Check sheet for the modelled part. Datum: model origin and axes. Units: mm. A direction names the side the tool comes from. Give positions to 0.01 mm unless a question says otherwise; leave off trailing zeros. Write each loop counter-clockwise with the first axis right and the second up, starting at its lowest first coordinate (ties: lowest second). Pieces come first, ordered by that corner, then holes. Notation, with made-up numbers: M 65.25,43.25 L 81.25,43.25 A24 ccw 81.25,64.25 Z; hole C -38.5,45 d6. An arc over 180 degrees is marked long. Write item = value, one per line. Start each with the question number.
1) Gauge pin test, flat ends, axial feed: pin 1 (0.7 mm diameter, centred on y = 0.5, z = -15.5, fed in from -X); pin 2 (0.8 mm diameter, centred on x = 34.5, y = 4, fed in from -Z); pin 3 (2.5 mm diameter, centred on y = 2.5, z = 2.5, fed in from -X). Record the tip position at first contact, or that the pin passes through.
2) Sectioned sample at B-B, the plane z = -7. Record the cut outline in (x, y), then the cut area to 3 significant figures.
3) Scan lines: L1, parallel to X at y = 1.6, z = 2.5; L2, parallel to X at y = 3.55, z = 7; L3, parallel to X at y = 0.9, z = -19.5. Record each from-to range of solid material in increasing order.
4) Sectioned sample at C-C, the plane x = -15.5. Record the cut outline in (y, z), then the cut area to 3 significant figures.
5) Sectioned sample at A-A, the plane x = 36.5. Record the cut outline in (y, z).
6) Set-up check for faces 4 (the face through (40.926, 3, 16)), 5 (the face through (37, 3, 4.458)), 6 (the face through (-36.274, 2, 3)), 7 (the face through (-32.274, 2, 3)): record each of +Z, -Z, +X, -X, +Y, -Y from which the full face is reachable in a straight line by a thin tool's end or side.
7) Draft check along Z on faces 1 (the face through (-2, 0, 4)), 2 (the face through (-41.324, 0.71, 14.295)), 3 (the face through (37, 3, 26.658)). Enter one of: pulls with the +Z half, pulls with the -Z half, needs draft (parallel to the pull), parting line crosses it, or undercut.
from build123d import *

# Parameters (mm, degrees)
SKETCH_1_W          = 85
SKETCH_1_H          = 56
EXTRUDE_1_DEPTH     = 1.4
FILLET_1_R          = 3
SKETCH_2_R          = 1.3
CUT_EXTRUDE_1_DEPTH = 1.5
SKETCH_7_R          = 3
CUT_EXTRUDE_4_DEPTH = 0.1
SKETCH_3_W          = 5
SKETCH_3_H          = 12.5
CUT_EXTRUDE_2_DEPTH = 1.5
FILLET_2_R          = 1
SKETCH_8_W          = 50
SKETCH_8_H          = 6.5
CUT_EXTRUDE_5_DEPTH = 54.614950043
FILLET_3_R          = 1
SKETCH_4_W          = 6.8
SKETCH_4_H          = 22
EXTRUDE_2_DEPTH     = 3.2
SKETCH_5_W          = 1.5
SKETCH_5_H          = 20.4
CUT_EXTRUDE_3_DEPTH = 1.8
SKETCH_6_W          = 4
SKETCH_6_H          = 12.5
EXTRUDE_3_DEPTH     = 2.2
SKETCH_10_R         = 2.85
EXTRUDE_4_DEPTH     = 1.4
SKETCH_9_R          = 1.85
CUT_EXTRUDE_6_DEPTH = 56.978914621
FILLET_4_R          = 1


with BuildPart() as part:
    # 草图1 → 凸台-拉伸1 (new body)
    with BuildSketch(Plane(origin=(0, 0, 0), x_dir=(1, 0, 0), z_dir=(0, 1, 0))):
        with Locations((-0.074300699, -4.558129371)):
            Rectangle(SKETCH_1_W, SKETCH_1_H)
    extrude(amount=EXTRUDE_1_DEPTH)

    # 圆角1
    fillet_1_edges = [part.edges().sort_by_distance(p)[0] for p in [
        (-42.574300699, 0.7, -23.441870629),
        (42.425699301, 0.7, -23.441870629),
        (42.425699301, 0.7, 32.558129371),
        (-42.574300699, 0.7, 32.558129371),
    ]]
    fillet(fillet_1_edges, radius=FILLET_1_R)

    # 草图2 → 切除-拉伸1 (cut)
    with BuildSketch(Plane(origin=(0, 1.4, 0), x_dir=(1, 0, 0), z_dir=(0, 1, 0))):
        with Locations(Location((-39.074300699, 19.941870629, 0), (0, 0, 270))):
            Circle(SKETCH_2_R)
        with Locations(Location((-39.074300699, -29.058129371, 0), (0, 0, 270))):
            Circle(SKETCH_2_R)
        with Locations(Location((18.925699301, -29.058129371, 0), (0, 0, 270))):
            Circle(SKETCH_2_R)
        with Locations(Location((18.925699301, 19.941870629, 0), (0, 0, 270))):
            Circle(SKETCH_2_R)
    extrude(amount=-CUT_EXTRUDE_1_DEPTH, mode=Mode.SUBTRACT)

    # 草图7 → 切除-拉伸4 (cut)
    with BuildSketch(Plane(origin=(0, 1.4, 0), x_dir=(1, 0, 0), z_dir=(0, 1, 0))):
        with Locations(Location((-39.074300699, 19.941870629, 0), (0, 0, 270))):
            Circle(SKETCH_7_R)
        with Locations(Location((18.925699301, 19.941870629, 0), (0, 0, 270))):
            Circle(SKETCH_7_R)
        with Locations(Location((-39.074300699, -29.058129371, 0), (0, 0, 270))):
            Circle(SKETCH_7_R)
        with Locations(Location((18.925699301, -29.058129371, 0), (0, 0, 270))):
            Circle(SKETCH_7_R)
    extrude(amount=-CUT_EXTRUDE_4_DEPTH, mode=Mode.SUBTRACT)

    # 草图3 → 切除-拉伸2 (cut)
    with BuildSketch(Plane(origin=(0, 1.4, 0), x_dir=(1, 0, 0), z_dir=(0, 1, 0))):
        with Locations((-40.074300699, -2.808129371)):
            Rectangle(SKETCH_3_W, SKETCH_3_H)
    extrude(amount=-CUT_EXTRUDE_2_DEPTH, mode=Mode.SUBTRACT)

    # 圆角2
    fillet_2_edges = [part.edges().sort_by_distance(p)[0] for p in [
        (-42.574300699, 0.7, 9.058129371),
        (-42.574300699, 0.7, -3.441870629),
        (-37.574300699, 0.7, -3.441870629),
        (-37.574300699, 0.7, 9.058129371),
    ]]
    fillet(fillet_2_edges, radius=FILLET_2_R)

    # 草图8 → 切除-拉伸5 (cut, through all)
    with BuildSketch(Plane(origin=(0, 1.4, 0), x_dir=(1, 0, 0), z_dir=(0, 1, 0))):
        with Locations((-10.074300699, 20.191870629)):
            Rectangle(SKETCH_8_W, SKETCH_8_H)
    extrude(amount=-CUT_EXTRUDE_5_DEPTH, mode=Mode.SUBTRACT)

    # 圆角3
    fillet_3_edges = [part.edges().sort_by_distance(p)[0] for p in [
        (-35.074300699, 0.7, -16.941870629),
        (-35.074300699, 0.7, -23.441870629),
        (14.925699301, 0.7, -23.441870629),
        (14.925699301, 0.7, -16.941870629),
    ]]
    fillet(fillet_3_edges, radius=FILLET_3_R)

    # 草图4 → 凸台-拉伸2 (add)
    with BuildSketch(Plane(origin=(0, 1.4, 0), x_dir=(1, 0, 0), z_dir=(0, 1, 0))):
        with Locations((37.525699301, 6.541870629)):
            Rectangle(SKETCH_4_W, SKETCH_4_H)
        with Locations((37.525699301, -15.658129371)):
            Rectangle(SKETCH_4_W, SKETCH_4_H)
    extrude(amount=EXTRUDE_2_DEPTH)

    # 草图5 → 切除-拉伸3 (cut)
    with BuildSketch(Plane(origin=(0, 4.6, 0), x_dir=(1, 0, 0), z_dir=(0, 1, 0))):
        with Locations((34.875699301, 6.541870629)):
            Rectangle(SKETCH_5_W, SKETCH_5_H)
        with Locations((34.875699301, -15.658129371)):
            Rectangle(SKETCH_5_W, SKETCH_5_H)
    extrude(amount=-CUT_EXTRUDE_3_DEPTH, mode=Mode.SUBTRACT)

    # 草图6 → 凸台-拉伸3 (add)
    with BuildSketch(Plane(origin=(0, 1.4, 0), x_dir=(1, 0, 0), z_dir=(0, 1, 0))):
        with Locations((-34.274300699, -2.808129371)):
            Rectangle(SKETCH_6_W, SKETCH_6_H)
    extrude(amount=EXTRUDE_3_DEPTH)

    # 草图10 → 凸台-拉伸4 (add)
    with BuildSketch(Plane(origin=(0, 1.4, 0), x_dir=(1, 0, 0), z_dir=(0, 1, 0))):
        with Locations((-42.574300699, 6.541870629)):
            Circle(SKETCH_10_R)
        with Locations((-42.574300699, -15.658129371)):
            Circle(SKETCH_10_R)
    extrude(amount=-EXTRUDE_4_DEPTH)

    # 草图9 → 切除-拉伸6 (cut, through all)
    with BuildSketch(Plane(origin=(0, 1.4, 0), x_dir=(1, 0, 0), z_dir=(0, 1, 0))):
        with Locations(Location((7.425699301, 6.541870629, 0), (0, 0, 270))):
            Circle(SKETCH_9_R)
        with Locations(Location((-4.574300699, 6.541870629, 0), (0, 0, 270))):
            Circle(SKETCH_9_R)
        with Locations(Location((-22.574300699, 6.541870629, 0), (0, 0, 270))):
            Circle(SKETCH_9_R)
        with Locations(Location((-22.574300699, -15.658129371, 0), (0, 0, 270))):
            Circle(SKETCH_9_R)
        with Locations(Location((-4.574300699, -15.658129371, 0), (0, 0, 270))):
            Circle(SKETCH_9_R)
        with Locations(Location((7.425699301, -15.658129371, 0), (0, 0, 270))):
            Circle(SKETCH_9_R)
        with Locations(Location((-42.574300699, 6.541870629, 0), (0, 0, 270))):
            Circle(SKETCH_9_R)
        with Locations(Location((-42.574300699, -15.658129371, 0), (0, 0, 270))):
            Circle(SKETCH_9_R)
    extrude(amount=-CUT_EXTRUDE_6_DEPTH, mode=Mode.SUBTRACT)

    # 圆角4
    fillet_4_edges = [part.edges().sort_by_distance(p)[0] for p in [
        (-42.255485289, 0.7, -3.70975892),
        (-42.574300699, 0.7, -9.391870629),
        (-42.574300699, 0.7, 12.808129371),
        (-42.574300699, 0.7, 18.508129371),
    ]]
    fillet(fillet_4_edges, radius=FILLET_4_R)


solid = part.part
Data:
q1.pin_1 = -42.57
q1.pin_2 = -17.54
q1.pin_3 = -37.57
q2.outline = M -45.39,0 L -44.37,0 L -44.37,1.4 L -45.39,1.4 Z; M -40.78,0 L -24.37,0 L -24.37,1.4 L -40.78,1.4 Z; M -20.78,0 L -6.37,0 L -6.37,1.4 L -20.78,1.4 Z; M -2.78,0 L 5.63,0 L 5.63,1.4 L -2.78,1.4 Z; M 9.22,0 L 42.43,0 L 42.43,1.4 L 40.93,1.4 L 40.93,4.6 L 35.63,4.6 L 35.63,2.8 L 34.13,2.8 L 34.13,1.4 L 9.22,1.4 Z
q2.area = 122 mm2
q3.L1 = -36.27 to -32.27, 34.13 to 40.93
q3.L2 = -36.27 to -32.27, 35.63 to 40.93
q3.L3 = -42.57 to -40.3, -37.85 to -35.07, 14.93 to 17.7, 20.15 to 42.43
q4.outline = M 0,-16.94 L 1.4,-16.94 L 1.4,32.56 L 0,32.56 Z
q4.area = 69.3 mm2
q5.outline = M 0,-23.44 L 1.4,-23.44 L 1.4,-17.54 L 4.6,-17.54 L 4.6,4.46 L 1.4,4.46 L 1.4,4.66 L 4.6,4.66 L 4.6,26.66 L 1.4,26.66 L 1.4,32.56 L 0,32.56 Z
q6.face_4 = +Z, -Z, +X, +Y
q6.face_5 = +X, +Y
q6.face_6 = +Z, -Z, -X, +Y
q6.face_7 = +Z, -Z, +Y
q7.face_1 = needs draft
q7.face_2 = undercut
q7.face_3 = pulls with the +Z half
